from build123d import *

# Parameters (mm, degrees)
SKETCH_1_W               = 150
SKETCH_1_H               = 38
EXTRUDE_1_DEPTH          = 9
SKETCH_2_R               = 1.3
CUT_EXTRUDE_1_DEPTH      = 8
PATTERN_LINEAR_1_COUNT   = 5
PATTERN_LINEAR_1_PITCH   = 21
MIRROR_1_COPY_1_SKETCH_R = 1.3
MIRROR_1_COPY_1_DEPTH    = 8
MIRROR_1_COPY_2_SKETCH_R = 1.3
MIRROR_1_COPY_2_DEPTH    = 8
MIRROR_1_COPY_3_SKETCH_R = 1.3
MIRROR_1_COPY_3_DEPTH    = 8
MIRROR_1_COPY_4_SKETCH_R = 1.3
MIRROR_1_COPY_4_DEPTH    = 8
CUT_EXTRUDE_2_REACH      = 79.891
SKETCH_3_R               = 2.5


with BuildPart() as part:
    # Sketch 1 → Extrude 1 (new body)
    with BuildSketch(Plane.XY):
        Rectangle(SKETCH_1_W, SKETCH_1_H)
    extrude(amount=EXTRUDE_1_DEPTH)

    # Sketch 2 → Cut-Extrude 1 (cut)
    with BuildSketch(Plane(origin=(0, 19, 0), x_dir=(1, 0, 0), z_dir=(0, 1, 0))):
        with Locations(Location((-42, -4.5, 0), (0, 0, 270))):
            Circle(SKETCH_2_R)
    cut_extrude_1 = extrude(amount=-CUT_EXTRUDE_1_DEPTH, mode=Mode.SUBTRACT)

    # Pattern Linear 1: Cut-Extrude 1 ×5
    with Locations(*[(i * PATTERN_LINEAR_1_PITCH, 0, 0) for i in range(1, PATTERN_LINEAR_1_COUNT)]):
        add(cut_extrude_1, mode=Mode.SUBTRACT)

    # Mirror 1: Cut-Extrude 1 across plane
    add(cut_extrude_1.mirror(Plane.ZX), mode=Mode.SUBTRACT)

    # Mirror 1 copy 1 sketch → Mirror 1 copy 1 (cut)
    with BuildSketch(Plane(origin=(21, -19, 0), x_dir=(1, 0, 0), z_dir=(0, -1, 0))):
        with Locations((-42, 4.5)):
            Circle(MIRROR_1_COPY_1_SKETCH_R)
    extrude(amount=-MIRROR_1_COPY_1_DEPTH, mode=Mode.SUBTRACT)

    # Mirror 1 copy 2 sketch → Mirror 1 copy 2 (cut)
    with BuildSketch(Plane(origin=(42, -19, 0), x_dir=(1, 0, 0), z_dir=(0, -1, 0))):
        with Locations((-42, 4.5)):
            Circle(MIRROR_1_COPY_2_SKETCH_R)
    extrude(amount=-MIRROR_1_COPY_2_DEPTH, mode=Mode.SUBTRACT)

    # Mirror 1 copy 3 sketch → Mirror 1 copy 3 (cut)
    with BuildSketch(Plane(origin=(63, -19, 0), x_dir=(1, 0, 0), z_dir=(0, -1, 0))):
        with Locations((-42, 4.5)):
            Circle(MIRROR_1_COPY_3_SKETCH_R)
    extrude(amount=-MIRROR_1_COPY_3_DEPTH, mode=Mode.SUBTRACT)

    # Mirror 1 copy 4 sketch → Mirror 1 copy 4 (cut)
    with BuildSketch(Plane(origin=(84, -19, 0), x_dir=(1, 0, 0), z_dir=(0, -1, 0))):
        with Locations((-42, 4.5)):
            Circle(MIRROR_1_COPY_4_SKETCH_R)
    extrude(amount=-MIRROR_1_COPY_4_DEPTH, mode=Mode.SUBTRACT)

    # Sketch 3 → Cut-Extrude 2 (cut, up to next)
    with BuildSketch(Plane.XY.offset(9), mode=Mode.PRIVATE) as cut_extrude_2_sk1:
        with Locations((-61, 0)):
            Circle(SKETCH_3_R)
    cut_extrude_2_tool1 = extrude(cut_extrude_2_sk1.sketch, amount=-CUT_EXTRUDE_2_REACH, mode=Mode.PRIVATE) & part.part
    # Sketch 3 → Cut-Extrude 2 (cut, up to next)
    with BuildSketch(Plane.XY.offset(9), mode=Mode.PRIVATE) as cut_extrude_2_sk2:
        with Locations((-43, 0)):
            Circle(SKETCH_3_R)
    cut_extrude_2_tool2 = extrude(cut_extrude_2_sk2.sketch, amount=-CUT_EXTRUDE_2_REACH, mode=Mode.PRIVATE) & part.part
    cut_extrude_2_1 = cut_extrude_2_tool1.solids().sort_by_distance((-61, 0, 9))[0]
    add(cut_extrude_2_1, mode=Mode.SUBTRACT)
    cut_extrude_2_2 = cut_extrude_2_tool2.solids().sort_by_distance((-43, 0, 9))[0]
    add(cut_extrude_2_2, mode=Mode.SUBTRACT)
    cut_extrude_2 = cut_extrude_2_1 + cut_extrude_2_2  # Cut-Extrude 2 as one shape, for the pattern or mirror that repeats it

    # Mirror 2: Cut-Extrude 2 across plane
    add(cut_extrude_2.mirror(Plane(origin=(0, 0, 0), x_dir=(0, 0, 1), z_dir=(1, 0, 0))), mode=Mode.SUBTRACT)


solid = part.part
Model file for the job. Use its own axes, mm. A direction names the side the tool comes from. Give positions to 0.01 mm unless a question says otherwise; leave off trailing zeros. Loops run counter-clockwise (first coordinate to the right, second up) from the corner with the lowest first, then second, coordinate; pieces in that order, holes last.
1) Flat gauge pins, fed straight in: pin 1 Ø0.8 at (x, z) = (-0.5, 4) entering from -Y; pin 2 Ø4.5 at (x, y) = (-61, 0) entering from +Z; pin 3 Ø2 at (x, z) = (-42, 4.5) entering from +Y. Where does each tip first touch, or does it go through?
2) Tool access for faces 5 (the flat face through (-1, 19, 3)), 6 (the flat face through (42, 11, 4)), 7 (the cylindrical face through (-22.03, -15.06, 3.71)): list every direction of +Z, -Z, +X, -X, +Y, -Y with a clear straight run to the whole face (end or side of a thin tool).
3) Saw through at C-C (x = -42). Write the cut outline in (y, z).
4) Pull direction X, two halves, no side cores. Call faces 1 (the flat face through (75, 0, 4)), 2 (the flat face through (-75, 0, 4)), 3 (the flat face through (21, -11, 5)), 4 (the flat face through (-1, 0, 9)): +X half, -X half, draft (parallel to the pull), parting line (faces both ways), or undercut.
5) Saw through at B-B (x = -61). Write the cut outline in (y, z).
6) Wall check: line 1 (Y direction, x = -61, z = 4.5); line 2 (X direction, y = 17, z = 4.5); line 3 (Y direction, x = -59.5, z = 0.75). Give the ranges that are in metal, low to high.
7) Saw through at A-A (x = 21). Write the cut outline in (y, z), plus the area to 3 significant figures.
Answer block:
1. pin 1: stops at y = -11
1. pin 2: passes through
1. pin 3: stops at y = 11
2. face 5: +Z, -Z, +X, -X, +Y
2. face 6: +Y
2. face 7: -Y
3. outline: (-19, 0) - (-2.29, 0) - (-2.29, 9) - (-19, 9) - (-19, 5.8) - (-11, 5.8) - (-11, 3.2) - (-19, 3.2) - close; (2.29, 0) - (19, 0) - (19, 3.2) - (11, 3.2) - (11, 5.8) - (19, 5.8) - (19, 9) - (2.29, 9) - close
4. face 1: +X half
4. face 2: -X half
4. face 3: undercut
4. face 4: draft
5. outline: (-19, 0) - (-2.5, 0) - (-2.5, 9) - (-19, 9) - close; (2.5, 0) - (19, 0) - (19, 9) - (2.5, 9) - close
6. line 1: y = -19 to -2.5, 2.5 to 19
6. line 2: x = -75 to -43.3, -40.7 to -22.3, -19.7 to -1.3, 1.3 to 19.7, 22.3 to 40.7, 43.3 to 75
6. line 3: y = -19 to -2, 2 to 19
7. outline: (-19, 0) - (19, 0) - (19, 3.2) - (11, 3.2) - (11, 5.8) - (19, 5.8) - (19, 9) - (-19, 9) - (-19, 5.8) - (-11, 5.8) - (-11, 3.2) - (-19, 3.2) - close
7. area: 300 mm2
